Work out the finished part from the listing and answer in its coordinate system (mm). Give positions to 0.01 mm unless a question says otherwise; leave off trailing zeros. Loops run counter-clockwise (first coordinate to the right, second up) from the corner with the lowest first, then second, coordinate; pieces in that order, holes last.
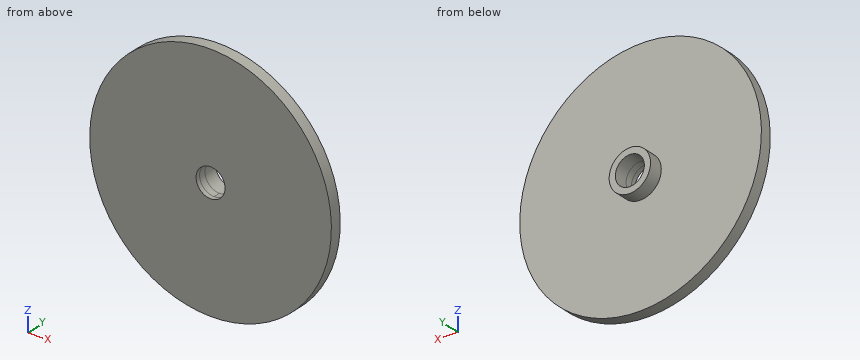
from build123d import *

# Parameters (mm, degrees)
SKETCH_1_R           = 3
SKETCH_1_R_2         = 2.1
EXTRUDE_1_DEPTH      = 3
EXTRUDE_2_DEPTH      = 0.65
EXTRUDE_2_DEPTH_BACK = 1
SKETCH_2_R           = 17.5
SKETCH_2_R_2         = 2.1


with BuildPart() as part:
    # ｽｹｯﾁ1 → ﾎﾞｽ - 押し出し1 (new body)
    with BuildSketch(Plane(origin=(0, 0, 0), x_dir=(1, 0, 0), z_dir=(0, 1, 0))):
        with Locations(Location((0, 0, 0), (0, 0, 270))):
            Circle(SKETCH_1_R)
        with Locations(Location((0, 0, 0), (0, 0, 270))):
            Circle(SKETCH_1_R_2, mode=Mode.SUBTRACT)
    extrude(amount=EXTRUDE_1_DEPTH)

    # ｽｹｯﾁ2 → ﾎﾞｽ - 押し出し2 (add, two sides: drawn at the far end of the back side and taken through both)
    with BuildSketch(Plane.XZ.offset(-EXTRUDE_2_DEPTH_BACK)):
        with Locations(Location((0, 0, 0), (0, 0, 270))):
            Circle(SKETCH_2_R)
        with Locations(Location((0, 0, 0), (0, 0, 270))):
            Circle(SKETCH_2_R_2, mode=Mode.SUBTRACT)
    extrude(amount=EXTRUDE_2_DEPTH + EXTRUDE_2_DEPTH_BACK)


solid = part.part
Item 1: Find section D-D, the plane z = 5. Write down the section's boundary in (x, y), plus the area to 3 significant figures.
Item 2: Find section C-C, the plane x = -14. Write down the section's boundary in (y, z), plus the area to 4 significant figures.
Item 3: Find section A-A, the plane z = 0. Write down the section's boundary in (x, y), plus the area to 3 significant figures.
Item 4: Flat-ended cylindrical pins translate along their axes: pin 1 Ø1.5 at (y, z) = (0, 13) entering from -X; pin 2 Ø1.5 at (x, y) = (13.5, 0.5) entering from -Z; pin 3 Ø1 at (y, z) = (0, 4.5) entering from -X. Find the tip coordinate at first contact, or state that the pin passes through.
Item 5: Find section B-B, the plane y = 1.4. Write down the section's boundary in (x, z), plus the area to 3 significant figures.
Item 6: Consider line 1 (X direction, y = 2.2, z = 0); line 2 (X direction, y = -0.3, z = 0). Determine where each line is inside the solid, lowest interval first.
Ans:
1. outline: (-16.77, -0.65) - (16.77, -0.65) - (16.77, 1) - (-16.77, 1) - close
1. area: 55.3 mm2
2. outline: (-0.65, -10.5) - (1, -10.5) - (1, 10.5) - (-0.65, 10.5) - close
2. area: 34.65 mm2
3. outline: (-17.5, -0.65) - (-2.1, -0.65) - (-2.1, 3) - (-3, 3) - (-3, 1) - (-17.5, 1) - close; (2.1, -0.65) - (17.5, -0.65) - (17.5, 1) - (3, 1) - (3, 3) - (2.1, 3) - close
3. area: 54.4 mm2
4. pin 1: stops at x = -12.5
4. pin 2: stops at z = -11.99
4. pin 3: stops at x = -17.04
5. outline: circle Ø6 at (0, 0); hole circle Ø4.2 at (0, 0)
5. area: 14.4 mm2
6. line 1: x = -3 to -2.1, 2.1 to 3
6. line 2: x = -17.5 to -2.1, 2.1 to 17.5
